from build123d import *

# Parameters (mm, degrees)
F0_R     = 1.25
F1_DEPTH = 10
F3_DEPTH = 5
F5_DEPTH = 2.6
F6_R     = 1.5
F7_DEPTH = 3
F8_DEPTH = 4.5
F9_SIZE  = 1
F10_SIZE = 1


with BuildPart() as f1:
    # F0 (on Top) → F1 (new body)
    with BuildSketch(Plane.XY):
        with BuildLine():
            Line((0, 9), (0, 0))
            Line((0, 0), (12.9, 0))
            ThreePointArc((12.9, 0), (8.4, 4.5), (12.9, 9))
            Line((12.9, 9), (0, 9))
        make_face()
        with Locations((3.9, 2.3)):
            Circle(F0_R, mode=Mode.SUBTRACT)
        with BuildLine():
            ThreePointArc((12.9, 9), (8.4, 4.5), (12.9, 0))
            Line((12.9, 0), (12.9, 1.6))
            ThreePointArc((12.9, 1.6), (10, 4.5), (12.9, 7.4))
            Line((12.9, 7.4), (12.9, 9))
        make_face()
        with BuildLine():
            Line((12.9, 1.6), (12.9, 0))
            ThreePointArc((12.9, 0), (16.0819805153, 1.3180194847), (17.4, 4.5))
            ThreePointArc((17.4, 4.5), (16.0819805153, 7.6819805153), (12.9, 9))
            Line((12.9, 9), (12.9, 7.4))
            ThreePointArc((12.9, 7.4), (14.9506096654, 6.5506096654), (15.8, 4.5))
            ThreePointArc((15.8, 4.5), (14.9506096654, 2.4493903346), (12.9, 1.6))
        make_face()
    extrude(amount=-F1_DEPTH)

    # F2 (on face) → F3 (cut)
    with BuildSketch(Plane.XY):
        Polygon((7.8917525037, 5.9926835701), (2.2893827112, 7.4938340317), (1.616453194, 4.9824268834), (7.2188229864, 3.4812764218), align=None)
    extrude(amount=-F3_DEPTH, mode=Mode.SUBTRACT)

    # F4 (on face) → F5 (cut, through all)
    with BuildSketch(Plane(origin=(2.0268180701, 7.5641880153, 0), x_dir=(0.9659258263, -0.2588190451, 0), z_dir=(-0.2588190451, -0.9659258263, 0))):
        Polygon((6.0718269188, -5.9743157806), (6.0718269188, -2.6256842194), (3.1718269188, -0.9513684387), (0.2718269188, -2.6256842194), (0.2718269188, -5.9743157806), (3.1718269188, -7.6486315613), align=None)
    extrude(amount=F5_DEPTH, mode=Mode.SUBTRACT)

    # F6 (on face) → F7 (cut)
    with BuildSketch(Plane(origin=(2.0268180701, 7.5641880153, 0), x_dir=(0.9659258263, -0.2588190451, 0), z_dir=(-0.2588190451, -0.9659258263, 0))):
        with Locations((3.1718269188, -4)):
            Circle(F6_R)
    extrude(amount=-F7_DEPTH, mode=Mode.SUBTRACT)

    # F6 (on face) → F8 (cut)
    with BuildSketch(Plane(origin=(2.0268180701, 7.5641880153, 0), x_dir=(0.9659258263, -0.2588190451, 0), z_dir=(-0.2588190451, -0.9659258263, 0))):
        with Locations((3.1718269188, -4)):
            Circle(F6_R)
    extrude(amount=F8_DEPTH, mode=Mode.SUBTRACT)

    # F9
    f9_edges = [f1.edges().sort_by_distance(p)[0] for p in [
        (0, 0, -5),
    ]]
    chamfer(f9_edges, length=F9_SIZE)

    # F10
    f10_edges = [f1.edges().sort_by_distance(p)[0] for p in [
        (0, 9, -5),
    ]]
    chamfer(f10_edges, length=F10_SIZE)


solid = f1.part
Work out the finished part from the listing and answer in its coordinate system (mm). A direction names the side the tool comes from. Coordinates: 2 decimals unless noted, no trailing zeros. Write each loop counter-clockwise with the first axis right and the second up, starting at its lowest first coordinate (ties: lowest second). Pieces come first, ordered by that corner, then holes. Notation, with made-up numbers: M 86.5,85.5 L 116.5,85.5 A19 cw 116.5,112.5 Z; hole C -12.75,63.5 d10. An arc over 180 degrees is marked long. Answer as CSV lines item,"result". Start each with the question number.
Item 1: Section D-D on z = -6.25 is taken. Write down the section's boundary in (x, y), and give its area (3 significant figures).
Item 2: Determine the mould class of faces 1 (the face through (9, 5, 0)), 2 (the face through (6.743, 7.383, -3.549)), 3 (the face through (0.5, 0.5, -4.9)), 4 (the face through (4.9, 3.35, -5.33)) for opening direction Z: released by +Z, released by -Z, zero draft, split by the parting line, or undercut.
Item 3: Section A-A on z = -2.25 is taken. Write down the section's boundary in (x, y), and give its area (3 significant figures).
Item 4: Consider L1, parallel to X at y = 5.75, z = -6.25; L2, parallel to Y at x = 3.9, z = -5.75; L3, parallel to X at y = 4.5, z = -9. Determine where each line is inside the solid, lowest interval first.
Item 5: A tool of negligible diameter and unlimited length cuts with its end or side. For faces 5 (the face through (6.14, 5.135, -6.823)), 6 (the face through (0.5, 8.5, -4.9)), from which of +Z, -Z, +X, -X, +Y, -Y can it reach the whole face along a straight path? Write none if from no direction.
Item 6: Section C-C on y = 2.3 is taken. Give the number of separate pieces and of enclosed holes in the cut face, and give its area (3 significant figures).
Item 7: Section B-B on z = -8.75 is taken. Write down the section's boundary in (x, y), and give its area (3 significant figures).
Checks:
1,outline,"M 0,1 L 1,0 L 12.9,0 A4.5 ccw 12.9,9 L 1,9 L 0,8 Z; hole M 2.08,4.86 L 6.76,3.6 L 7.43,6.12 L 2.75,7.37 Z; hole C 3.9,2.3 d2.5; hole C 12.9,4.5 d5.8"
1,area,"103 mm²"
2,face 1,"released by +Z"
2,face 2,"undercut"
2,face 3,"zero draft"
2,face 4,"undercut"
3,outline,"M 0,1 L 1,0 L 12.9,0 A4.5 ccw 12.9,9 L 1,9 L 0,8 Z; hole M 1.62,4.98 L 7.22,3.48 L 7.89,5.99 L 2.29,7.49 Z; hole C 3.9,2.3 d2.5; hole C 12.9,4.5 d5.8"
3,area,"100 mm²"
4,L1,"x = 0 to 2.32, 7.33 to 10.28, 15.52 to 17.22"
4,L2,"y = 0 to 1.05, 3.55 to 4.37, 7.06 to 9"
4,L3,"x = 0 to 10, 15.8 to 17.4"
5,face 5,"+Z"
5,face 6,"+Z, -Z, -X, +Y"
6,separate pieces,"3"
6,enclosed holes,"0"
6,area,"105 mm²"
7,outline,"M 0,1 L 1,0 L 12.9,0 A4.5 ccw 12.9,9 L 1,9 L 0,8 Z; hole C 3.9,2.3 d2.5; hole C 12.9,4.5 d5.8"
7,area,"116 mm²"
